The model under review builds one solid part; all positions refer to its coordinate system, in mm. A direction names the side the tool comes from. Give positions to 0.01 mm unless a question says otherwise; leave off trailing zeros. Order: outer loops, then holes, each group sorted by start corner. A loop starts at its lowest first (then second) coordinate and runs counter-clockwise, first axis right, second up. Notation, with made-up numbers: (45.25, 7.5) - (77.25, 7.5) arc R32 ccw to (77.25, 33.5) - close; hole circle Ø8 at (86.25, 65.25). An arc over 180 degrees is marked (long way). Use CSV: the item, a comma, the result in double quotes.
```python
from build123d import *

# Parameters (mm, degrees)
SKETCH_R           = 1.5
PAD_DEPTH          = 3
PAD001_DEPTH       = 3
POLARPATTERN_COUNT = 4
FILLET_R           = 0.3
FILLET001_R        = 0.5
FILLET002_R        = 0.3
FILLET003_R        = 0.3
FILLET004_R        = 0.3


with BuildPart() as part:
    # Sketch → Pad (new body)
    with BuildSketch(Plane.XY):
        with BuildLine():
            Line((-13.555442, 8.5), (-3.039737, 22.6))
            ThreePointArc((3.039737, 22.6), (0, 24), (-3.039737, 22.6))
            Line((3.039737, 22.6), (13.555442, 8.5))
            ThreePointArc((-13.555442, 8.5), (0, -16), (13.555442, 8.5))
        make_face()
        with Locations((0, 20)):
            Circle(SKETCH_R, mode=Mode.SUBTRACT)
    extrude(amount=-PAD_DEPTH)

    # Sketch001 (on Face6 of Pad) → Pad001 (join)
    with BuildSketch(Plane.XY):
        with BuildLine():
            Line((-2.76, 5.42), (2.76, 5.42))
            Line((2.76, 5.42), (7.92188, 10.58188))
            ThreePointArc((7.92188, 10.58188), (6.158918, 11.696157), (4.242641, 12.519279))
            Line((4.242641, 12.519279), (0, 8.276638))
            Line((0, 8.276638), (-4.242641, 12.519279))
            ThreePointArc((-4.242641, 12.519279), (-6.158918, 11.696157), (-7.92188, 10.58188))
            Line((-7.92188, 10.58188), (-2.76, 5.42))
        make_face()
    pad001 = extrude(amount=PAD001_DEPTH)

    # PolarPattern: Pad001 ×4 about axis
    polarpattern_axis = Axis((0, 0, 0), (0, 0, 1))
    for i in range(1, POLARPATTERN_COUNT):
        add(pad001.rotate(polarpattern_axis, i * 360 / POLARPATTERN_COUNT))

    # Fillet
    fillet_edges = [part.edges().sort_by_distance(p)[0] for p in [
        (-4.242641, 12.519279, 1.5),
        (0, 8.276638, 1.5),
        (4.242641, 12.519279, 1.5),
        (7.92188, 10.58188, 1.5),
        (2.76, 5.42, 1.5),
        (-2.76, 5.42, 1.5),
        (-7.92188, 10.58188, 1.5),
    ]]
    fillet(fillet_edges, radius=FILLET_R)

    # Fillet001
    fillet001_edges = [part.edges().sort_by_distance(p)[0] for p in [
        (-8.297589, 15.55, -3),
        (0, -16, -3),
        (8.297589, 15.55, -3),
        (0, 24, -3),
        (-1.5, 20, -3),
    ]]
    fillet(fillet001_edges, radius=FILLET001_R)

    # Fillet002
    fillet002_edges = [part.edges().sort_by_distance(p)[0] for p in [
        (-10.58188, 7.92188, 1.5),
        (-5.42, 2.76, 1.5),
        (-5.42, -2.76, 1.5),
        (-10.58188, -7.92188, 1.5),
        (-12.519279, -4.242641, 1.5),
        (-12.519279, 4.242641, 1.5),
        (-8.276638, 0, 1.5),
    ]]
    fillet(fillet002_edges, radius=FILLET002_R)

    # Fillet003
    fillet003_edges = [part.edges().sort_by_distance(p)[0] for p in [
        (-7.92188, -10.58188, 1.5),
        (-4.242641, -12.519279, 1.5),
        (4.242641, -12.519279, 1.5),
        (7.92188, -10.58188, 1.5),
        (0, -8.276638, 1.5),
        (-2.76, -5.42, 1.5),
        (2.76, -5.42, 1.5),
    ]]
    fillet(fillet003_edges, radius=FILLET003_R)

    # Fillet004
    fillet004_edges = [part.edges().sort_by_distance(p)[0] for p in [
        (10.58188, -7.92188, 1.5),
        (12.519279, -4.242641, 1.5),
        (12.519279, 4.242641, 1.5),
        (10.58188, 7.92188, 1.5),
        (8.276638, 0, 1.5),
        (5.42, -2.76, 1.5),
        (5.42, 2.76, 1.5),
    ]]
    fillet(fillet004_edges, radius=FILLET004_R)


solid = part.part
```
Item 1: Clearance check with flat-ended pins moving along their axes: pin 1 (2.5 mm diameter, centred on x = -0.5, z = 2, fed in from +Y); pin 2 (2.5 mm diameter, centred on y = -0.5, z = 2, fed in from +X); pin 3 (1.5 mm diameter, centred on y = -11, z = -1.5, fed in from +X). State where each tip first meets the part, or that it passes through.
Results list:
pin 1,"stops at y = 10.03"
pin 2,"stops at x = 10.03"
pin 3,"stops at x = 12.29"
Item 2: Mouldability with a two-part tool opening along X and no side actions: class faces 4 (the face through (8.257, 15.366, -2.85)), 5 (the face through (-7.95, -5.29, 1.48)), 6 (the face through (0, 8, 3)), 7 (the face through (-6.11, -11.72, 1.48)) as pulls with the +X half, pulls with the -X half, needs draft (parallel to the pull), parting line crosses it, or undercut.
Results list:
face 4,"pulls with the +X half"
face 5,"undercut"
face 6,"needs draft"
face 7,"pulls with the -X half"
Item 3: Take a section at A-A, the plane z = -1.05. Give the boundary of the cut face in (x, y), and give its area (3 significant figures).
Results list:
outline,"(-13.56, 8.5) arc R16 ccw (long way) to (13.56, 8.5) - (3.04, 22.6) arc R4 ccw to (-3.04, 22.6) - close; hole circle Ø3 at (0, 20)"
area,"894 mm2"
Item 4: Tool access review of faces 1 (the face through (-6.063, 11.746, 1.479)), 2 (the face through (-2.188, -10.465, 1.479)), 3 (the face through (-2.134, 10.41, 1.479)): name each direction out of +Z, -Z, +X, -X, +Y, -Y from which nothing blocks a thin tool from reaching the whole face with its end or side.
Results list:
face 1,"+Z, -X, +Y"
face 2,"+Z, -Y"
face 3,"+Z, +Y"
Item 5: Wall thickness on L1, parallel to Y at x = 0, z = -1.8; L2, parallel to Z at x = 2, y = 18.5; L3, parallel to Y at x = 9, z = 1.05: over which ranges is each line inside the solid? List them lowest first.
Results list:
L1,"y = -16 to 18.5, 21.5 to 24"
L2,"z = -3 to 0"
L3,"y = -6.34 to -0.72, 0.72 to 6.34"
